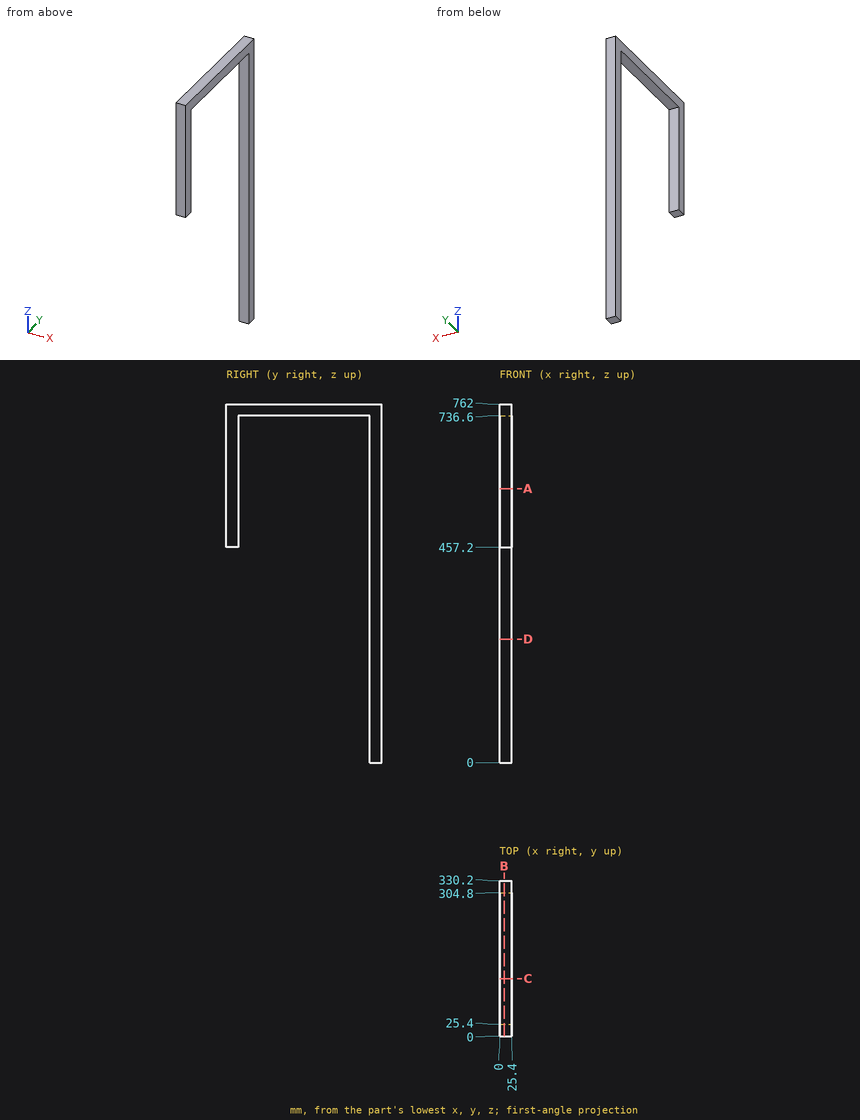
Verification items for this drawing (mm, ordinates from the low corner). Coordinates: 2 decimals unless noted, no trailing zeros. Loops run counter-clockwise (first coordinate to the right, second up) from the corner with the lowest first, then second, coordinate; pieces in that order, holes last. Notation, with made-up numbers: (-6, 73) - (22, 73) arc R7 ccw to (22, 77) - close; hole circle Ø5 at (-23.75, 79). An arc over 180 degrees is marked (long way). Use one line per item in the form item = value. Start each with the question number.
Item 1: Thickness scan on probe 1 along Y at (x, z) = (7.5, 505.5); probe 2 along Y at (x, z) = (17, 121); probe 3 along Z at (x, y) = (16, 211.5). Record the ranges inside material, lowest first.
Item 2: Section check B-B, the plane x = 9.25. Enter the section's corners in (y, z).
Item 3: Section check A-A, the plane z = 582. Enter the section's corners in (x, y), and give its area (3 significant figures).
Item 4: Section check D-D, the plane z = 262.5. Enter the section's corners in (x, y).
Item 5: Section check C-C, the plane y = 122. Enter the section's corners in (x, z).
Item 6: Gauge pin test, flat ends, axial feed: pin 1 (12.5 mm diameter, centred on x = 7.5, y = 11, fed in from -Z); pin 2 (5 mm diameter, centred on x = 21, z = 153, fed in from -Y); pin 3 (4 mm diameter, centred on x = 5.5, y = 234.5, fed in from -Z). Record the tip position at first contact, or that the pin passes through.
Computed:
q1.probe_1 = 0 to 25.4, 304.8 to 330.2
q1.probe_2 = 304.8 to 330.2
q1.probe_3 = 736.6 to 762
q2.outline = (0, 457.2) - (25.4, 457.2) - (25.4, 736.6) - (304.8, 736.6) - (304.8, 0) - (330.2, 0) - (330.2, 762) - (0, 762) - close
q3.outline = (0, 0) - (25.4, 0) - (25.4, 25.4) - (0, 25.4) - close; (0, 304.8) - (25.4, 304.8) - (25.4, 330.2) - (0, 330.2) - close
q3.area = 1,290 mm2
q4.outline = (0, 304.8) - (25.4, 304.8) - (25.4, 330.2) - (0, 330.2) - close
q5.outline = (0, 736.6) - (25.4, 736.6) - (25.4, 762) - (0, 762) - close
q6.pin_1 = 457.2
q6.pin_2 = 304.8
q6.pin_3 = 736.6
